Check sheet for the modelled part. Datum: model origin and axes. Units: mm. A direction names the side the tool comes from. Coordinates: 2 decimals unless noted, no trailing zeros. Write each loop counter-clockwise with the first axis right and the second up, starting at its lowest first coordinate (ties: lowest second). Pieces come first, ordered by that corner, then holes. Notation, with made-up numbers: (-27, 39) -> (21, 39) arc R20 cw to (21, 70) -> close; hole circle Ø11 at (-29, 76.25). An arc over 180 degrees is marked (long way). Put each result on its own line as item: value.
```python
from build123d import *

# Parameters (mm, degrees)
SZKIC1_W                    = 25.4
SZKIC1_H                    = 5.8
DODANIE_WYCI_GNI_CIE2_DEPTH = 3.4
SZKIC3_W                    = 0.64
SZKIC3_H                    = 0.643583424
WYTNIJ_WYCI_GNI_CIE1_DEPTH  = 3.4
SZKIC5_W                    = 5.8
SZKIC5_H                    = 3.4
DODANIE_WYCI_GNI_CIE3_DEPTH = 1
SZKIC6_W                    = 5.8
SZKIC6_H                    = 3.4
DODANIE_WYCI_GNI_CIE4_DEPTH = 1
SZKIC7_W                    = 27.4
SZKIC7_H                    = 5.8
SZKIC7_W_2                  = 25.404799249
SZKIC7_H_2                  = 3.8
DODANIE_WYCI_GNI_CIE6_DEPTH = 8.1
SZKIC8_W                    = 1
SZKIC8_H                    = 1
SZKIC8_W_2                  = 0.995200751
SZKIC8_H_2                  = 0.995200751
WYTNIJ_WYCI_GNI_CIE3_DEPTH  = 3
ZAOKR_GLENIE1_R             = 0.5


with BuildPart() as part:
    # Szkic1 → Dodanie-wyciągnięcie2 (new body)
    with BuildSketch(Plane(origin=(0, 0, 0), x_dir=(1, 0, 0), z_dir=(0, 1, 0))):
        Rectangle(SZKIC1_W, SZKIC1_H)
    extrude(amount=DODANIE_WYCI_GNI_CIE2_DEPTH)

    # Szkic3 → Wytnij-wyciągnięcie1 (cut)
    with BuildSketch(Plane(origin=(0, 3.4, 0), x_dir=(1, 0, 0), z_dir=(0, 1, 0))):
        with Locations((-11.43, 0)):
            Rectangle(SZKIC3_W, SZKIC3_H)
        with Locations((-8.89, 0)):
            Rectangle(SZKIC3_W, SZKIC3_H)
        with Locations((-6.35, 0)):
            Rectangle(SZKIC3_W, SZKIC3_H)
        with Locations((-3.81, 0)):
            Rectangle(SZKIC3_W, SZKIC3_H)
        with Locations((-1.27, 0)):
            Rectangle(SZKIC3_W, SZKIC3_H)
        with Locations((1.27, 0)):
            Rectangle(SZKIC3_W, SZKIC3_H)
        with Locations((3.81, 0)):
            Rectangle(SZKIC3_W, SZKIC3_H)
        with Locations((6.35, 0)):
            Rectangle(SZKIC3_W, SZKIC3_H)
        with Locations((8.89, 0)):
            Rectangle(SZKIC3_W, SZKIC3_H)
        with Locations((11.43, 0)):
            Rectangle(SZKIC3_W, SZKIC3_H)
    extrude(amount=-WYTNIJ_WYCI_GNI_CIE1_DEPTH, mode=Mode.SUBTRACT)

    # Szkic5 → Dodanie-wyciągnięcie3 (add)
    with BuildSketch(Plane.ZY.offset(12.7)):
        with Locations((0, 1.7)):
            Rectangle(SZKIC5_W, SZKIC5_H)
    extrude(amount=DODANIE_WYCI_GNI_CIE3_DEPTH)

    # Szkic6 → Dodanie-wyciągnięcie4 (add)
    with BuildSketch(Plane(origin=(12.7, 0, 0), x_dir=(0, 0, -1), z_dir=(1, 0, 0))):
        with Locations((0, 1.7)):
            Rectangle(SZKIC6_W, SZKIC6_H)
    extrude(amount=DODANIE_WYCI_GNI_CIE4_DEPTH)

    # Szkic7 → Dodanie-wyciągnięcie6 (add)
    with BuildSketch(Plane(origin=(0, 3.4, 0), x_dir=(1, 0, 0), z_dir=(0, 1, 0))):
        Rectangle(SZKIC7_W, SZKIC7_H)
        with Locations((-0.002399624, 0)):
            Rectangle(SZKIC7_W_2, SZKIC7_H_2, mode=Mode.SUBTRACT)
    extrude(amount=DODANIE_WYCI_GNI_CIE6_DEPTH)

    # Szkic8 → Wytnij-wyciągnięcie3 (cut)
    with BuildSketch(Plane(origin=(0, 11.5, 0), x_dir=(1, 0, 0), z_dir=(0, 1, 0))):
        with Locations((12.2, 2.4)):
            Rectangle(SZKIC8_W, SZKIC8_H)
        with Locations((13.2, 1.4)):
            Rectangle(SZKIC8_W, SZKIC8_H)
        with Locations((13.2, -1.4)):
            Rectangle(SZKIC8_W, SZKIC8_H)
        with Locations((12.2, -2.4)):
            Rectangle(SZKIC8_W, SZKIC8_H)
        with Locations((-12.204799249, -2.4)):
            Rectangle(SZKIC8_W, SZKIC8_H)
        with Locations((-13.202399624, -1.402399625)):
            Rectangle(SZKIC8_W_2, SZKIC8_H_2)
        with Locations((-13.202399624, 1.402399625)):
            Rectangle(SZKIC8_W_2, SZKIC8_H_2)
        with Locations((-12.204799249, 2.4)):
            Rectangle(SZKIC8_W, SZKIC8_H)
    extrude(amount=-WYTNIJ_WYCI_GNI_CIE3_DEPTH, mode=Mode.SUBTRACT)

    # Zaokrąglenie1
    zaokr_glenie1_edges = [part.edges().sort_by_distance(p)[0] for p in [
        (-13.202399624, 8.5, -0.904799249),
        (-13.202399624, 8.5, 0.904799249),
        (13.2, 8.5, 0.9),
        (13.2, 8.5, -0.9),
        (11.7, 8.5, -2.4),
        (11.7, 8.5, 2.4),
        (-11.704799249, 8.5, 2.4),
        (-11.704799249, 8.5, -2.4),
    ]]
    fillet(zaokr_glenie1_edges, radius=ZAOKR_GLENIE1_R)


solid = part.part
```
Q1. Cross-section at A-A (x = -3.75). Record the cut outline in (y, z).
Recorded:
outline: (0, -2.9) -> (11.5, -2.9) -> (11.5, -1.9) -> (3.4, -1.9) -> (3.4, -0.32) -> (0, -0.32) -> close; (0, 0.32) -> (3.4, 0.32) -> (3.4, 1.9) -> (11.5, 1.9) -> (11.5, 2.9) -> (0, 2.9) -> close
Q2. Material ranges on line 1 along Z through (x, y) = (-8.75, 10.5); line 2 along X through (y, z) = (10.75, 0.45); line 3 along Y through (x, z) = (1.75, -1.75), recorded low to high.
Recorded:
line 1: z = -2.9 to -1.9, 1.9 to 2.9
line 2: x = -13.7 to -12.7, 12.7 to 13.7
line 3: y = 0 to 3.4
Q3. Cross-section at C-C (y = 5.5). Record the cut outline in (x, z), plus the area to 3 significant figures.
Recorded:
outline: (-13.7, -2.9) -> (13.7, -2.9) -> (13.7, 2.9) -> (-13.7, 2.9) -> close; hole (-12.7, -1.9) -> (12.7, -1.9) -> (12.7, 1.9) -> (-12.7, 1.9) -> close
area: 62.4 mm2
Q4. Tool access check on faces 4 (the flat face through (0, 7, 1.9)), 5 (the flat face through (13, 11.5, 0)), 6 (the flat face through (-12.705, 10, -2.4)), 7 (the flat face through (13, 10, -1.9)). Record the directions out of +Z, -Z, +X, -X, +Y, -Y that give a thin tool (end or side, any length) a straight path to the whole face; none if there is none.
Recorded:
face 4: +Y
face 5: +Z, -Z, +X, -X, +Y
face 6: +Z, -Z, +Y
face 7: +X, -X, +Y
Q5. Cross-section at D-D (z = -2.45). Record the cut outline in (x, y).
Recorded:
outline: (-13.7, 0) -> (13.7, 0) -> (13.7, 11.5) -> (12.7, 11.5) -> (12.7, 8.5) -> (12.2, 8.5) arc R0.5 cw to (11.7, 9) -> (11.7, 11.5) -> (-11.7, 11.5) -> (-11.7, 9) arc R0.5 cw to (-12.2, 8.5) -> (-12.7, 8.5) -> (-12.7, 11.5) -> (-13.7, 11.5) -> close
Q6. Mould release check, pull along X, two halves, no side actions. Record for faces 1 (the flat face through (-12.705, 10, 2.4)), 2 (the flat face through (-0.2, 11.5, -2.4)), 3 (the flat face through (13.7, 6, 0)): released by +X, released by -X, zero draft, split by the parting line, or undercut.
Recorded:
face 1: undercut
face 2: zero draft
face 3: released by +X
Q7. Cross-section at B-B (y = 11.25). State how many separate pieces and enclosed holes the cut face has, plus the area to 3 significant figures.
Recorded:
separate pieces: 8
enclosed holes: 0
area: 54.4 mm2
